Could you check a few things on this drawing? It's one solid part, dimensions in mm from its lowest x, y, z. A direction names the side the tool comes from. Give positions to 0.01 mm unless a question says otherwise; leave off trailing zeros. Loops run counter-clockwise (first coordinate to the right, second up) from the corner with the lowest first, then second, coordinate; pieces in that order, holes last. Notation, with made-up numbers: M 75,-18 L 124,-18 A23 cw 124,-9 Z; hole C 38.25,-12.5 d6. An arc over 180 degrees is marked long. Answer in a Markdown table with one row per item. Add a question column.
1. I need wall thicknesses on line 1 along X through (y, z) = (2.75, 1.9); line 2 along Y through (x, z) = (42.5, 0.5) (3 decimals); line 3 along X through (y, z) = (4.25, 3.7). Which ranges of each line are inside material? Lowest first, please. Write a range as from..to.
2. If we section it at A-A on y = 3.5: List the corners of the cut face in (x, z) for me (3 decimals).
3. If we section it at D-D on x = 2.5: List the corners of the cut face in (y, z) for me (3 decimals).
4. Which directions (+Z, -Z, +X, -X, +Y, -Y) give clear straight access to the entire face, cutting with the end or side of a thin tool? Please do the marked faces 1 and 2.
5. I'm going to push a flat-ended pin straight in: pin 1 Ø2.5 at (y, z) = (3, 3.5) entering from +X. Where does the tip first touch, or does it pass through?
6. If we section it at C-C on z = 0.8: List the corners of the cut face in (x, y) for me (3 decimals), then the cut area to 3 significant figures.
7. If we section it at B-B on z = 4.3: List the corners of the cut face in (x, y) for me (3 decimals), then the cut area to 3 significant figures.
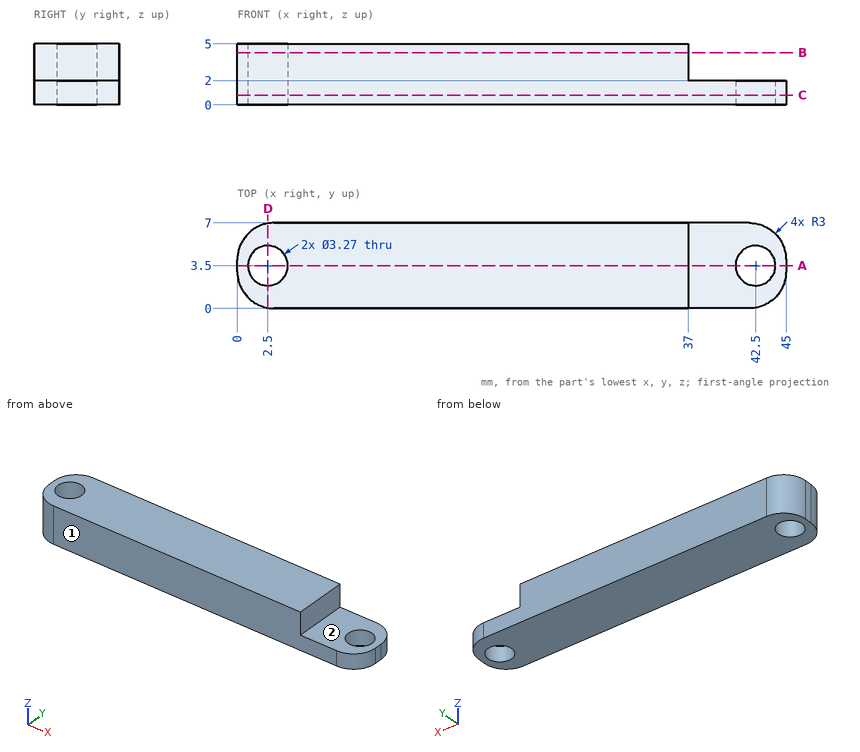
Results:
| question | item | result |
|---|---|---|
| 1 | line 1 | 0.01..1.05, 3.95..41.05, 43.95..44.99 |
| 1 | line 2 | 0.042..1.865, 5.135..6.958 |
| 1 | line 3 | 0.01..1.05, 3.95..37 |
| 2 | outline | M 0,0 L 0.865,0 L 0.865,5 L 0,5 Z; M 4.135,0 L 40.865,0 L 40.865,2 L 37,2 L 37,5 L 4.135,5 Z; M 44.135,0 L 45,0 L 45,2 L 44.135,2 Z |
| 3 | outline | M 0.042,0 L 1.865,0 L 1.865,5 L 0.042,5 Z; M 5.135,0 L 6.958,0 L 6.958,5 L 5.135,5 Z |
| 4 | face 1 | +Z, -Z, +X, -X, -Y |
| 4 | face 2 | +Z, +X, +Y, -Y |
| 5 | pin 1 | x = 37 |
| 6 | outline | M 0,3 A3 ccw 3,0 L 42,0 A3 ccw 45,3 L 45,4 A3 ccw 42,7 L 3,7 A3 ccw 0,4 Z; hole C 2.5,3.5 d3.27; hole C 42.5,3.5 d3.27 |
| 6 | area | 290 mm2 |
| 7 | outline | M 0,3 A3 ccw 3,0 L 37,0 L 37,7 L 3,7 A3 ccw 0,4 Z; hole C 2.5,3.5 d3.27 |
| 7 | area | 247 mm2 |
